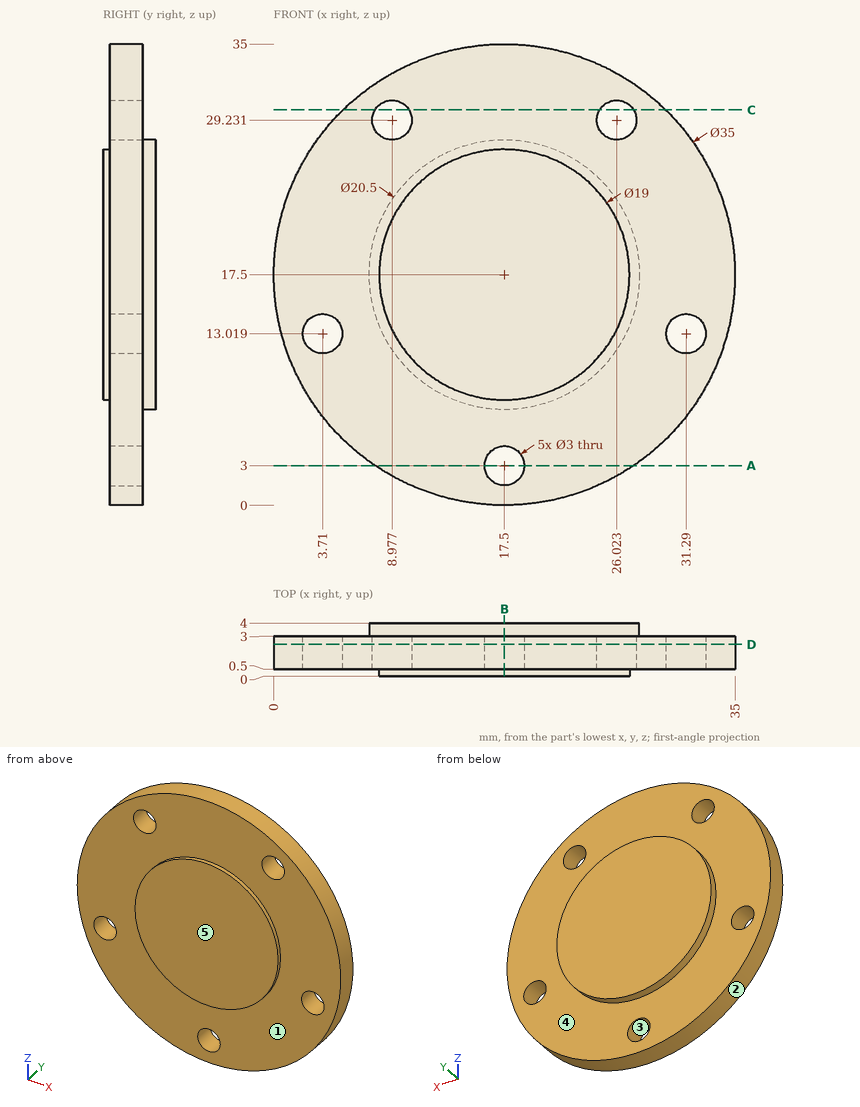
Answer from the drawing. Dimensions are ordinates in mm from the lowest x, y and z of the part. A direction names the side the tool comes from. Round coordinates to 2 decimals unless told otherwise and drop trailing zeros. Order: outer loops, then holes, each group sorted by start corner. A loop starts at its lowest first (then second) coordinate and runs counter-clockwise, first axis right, second up.
1) Straight lines are drawn through the part: L1, parallel to X at y = 2.95, z = 12.5; L2, parallel to Y at x = 5, z = 9; L3, parallel to Z at x = 17.5, y = 2.35. For each, find the intervals that lie inside material, in ascending order.
2) For the marked faces 4 and 5, determine the directions among +Z, -Z, +X, -X, +Y, -Y from which every point of the face is accessible in a straight line to the end or side of a thin tool.
3) Flat-ended cylindrical pins translate along their axes: pin 1 (1 mm diameter, centred on y = 2.5, z = 10, fed in from -X); pin 2 (4 mm diameter, centred on x = 8.98, z = 29.23, fed in from -Y); pin 3 (4 mm diameter, centred on x = 3.71, z = 13.02, fed in from +Y). Find the tip coordinate at first contact, or state that the pin passes through.
4) The mould has two halves that part along Z. Classify the marked faces 1, 2 and 3: released by +Z, released by -Z, zero draft, split by the parting line, or undercut.
5) The part is cut by section D-D on y = 2.4. Write down the section's boundary in (x, z), plus the area to 3 significant figures.
6) The part is cut by section A-A on z = 3. Write down the section's boundary in (x, y), plus the area to 3 significant figures.
7) The part is cut by section B-B on x = 17.5. Write down the section's boundary in (y, z).
8) The part is cut by section C-C on z = 30. Write down the section's boundary in (x, y) (1 decimal).
Resolved:
1. L1: x = 0.73 to 2.3, 5.12 to 29.88, 32.7 to 34.27
1. L2: y = 0.5 to 3
1. L3: z = 0 to 1.5, 4.5 to 35
2. face 4: +Y
2. face 5: +Z, -Z, +X, -X, -Y
3. pin 1: stops at x = 1.46
3. pin 2: stops at y = 0.5
3. pin 3: stops at y = 3
4. face 1: zero draft
4. face 2: split by the parting line
4. face 3: undercut
5. outline: circle Ø35 at (17.5, 17.5); hole circle Ø3 at (3.71, 13.02); hole circle Ø3 at (8.98, 29.23); hole circle Ø3 at (17.5, 3); hole circle Ø3 at (26.02, 29.23); hole circle Ø3 at (31.29, 13.02)
5. area: 927 mm2
6. outline: (7.7, 0.5) - (16, 0.5) - (16, 3) - (7.7, 3) - close; (19, 0.5) - (27.3, 0.5) - (27.3, 3) - (19, 3) - close
6. area: 41.5 mm2
7. outline: (0, 8) - (0.5, 8) - (0.5, 4.5) - (3, 4.5) - (3, 7.25) - (4, 7.25) - (4, 27.75) - (3, 27.75) - (3, 35) - (0.5, 35) - (0.5, 27) - (0, 27) - close; (0.5, 0) - (3, 0) - (3, 1.5) - (0.5, 1.5) - close
8. outline: (5.3, 0.5) - (7.7, 0.5) - (7.7, 3) - (5.3, 3) - close; (10.3, 0.5) - (24.7, 0.5) - (24.7, 3) - (10.3, 3) - close; (27.3, 0.5) - (29.7, 0.5) - (29.7, 3) - (27.3, 3) - close
